For this review, take the finished solid that the model builds, in its own axes (mm). A direction names the side the tool comes from. Coordinates: 2 decimals unless noted, no trailing zeros. Write each loop counter-clockwise with the first axis right and the second up, starting at its lowest first coordinate (ties: lowest second). Pieces come first, ordered by that corner, then holes. Notation, with made-up numbers: (86, -32.75) - (121, -32.75) arc R16 ccw to (121, -26.75) - close; hole circle Ø2 at (39, 82.5). An arc over 180 degrees is marked (long way). Use one line per item in the form item = value. Start each with the question number.
1) For L1, parallel to Y at x = -1.5, z = 5.5; L2, parallel to X at y = 6.25, z = 32; L3, parallel to Y at x = 8, z = 9, list the stretches that pass through material, from the lowest coordinate up. Write a range as from..to.
2) Insertion check: P1, Ø10.5, axis at x = -17.5, z = 12.5, coming from the -Y side; P2, Ø4, axis at x = -37.5, y = 2.5, coming from the -Z side; P3, Ø10, axis at x = -35.5, z = 8.5, coming from the -Y side. Each pin has a flat end and moves straight along its axis. Give the tip position at first contact, or say it passes through.
3) We need section B-B (x = -9.5). Give the boundary of the cut face in (y, z).
4) We need section A-A (y = 2). Give the boundary of the cut face in (x, z).
5) Mouldability with a two-part tool opening along X and no side actions: class faces 4 (the cylindrical face through (-38.185, -10.06, 17.578)), 5 (the flat face through (-9, 7.62, 18)), 6 (the flat face through (8, -8, 0)) as pulls with the +X half, pulls with the -X half, needs draft (parallel to the pull), parting line crosses it, or undercut.
6) We need section D-D (y = -5.5). Give the boundary of the cut face in (x, z), plus the area to 3 significant figures.
7) We need section C-C (x = 3). Give the boundary of the cut face in (y, z), plus the area to 3 significant figures.
8) Tool access review of faces 1 (the flat face through (-8, -7.62, 18)), 2 (the flat face through (-34, -6.35, 8)), 3 (the flat face through (5.17, 0.11, 17.58)): name each direction out of +Z, -Z, +X, -X, +Y, -Y from which nothing blocks a thin tool from reaching the whole face with its end or side.
```python
from build123d import *

# Parameters (mm, degrees)
F1_DEPTH      = 34.671
F2_R          = 2.54
F5_DEPTH      = 59.1859747542
F7_DEPTH      = 6.35
F7_DEPTH_BACK = 6.35


with BuildPart() as f1:
    # F0 (on Top) → F1 (new body)
    with BuildSketch(Plane.XY):
        Polygon((38.89375, 12.192), (-38.89375, 10.795), (-38.89375, -10.795), (38.89375, -12.192), align=None)
    extrude(amount=F1_DEPTH)

    # F2
    f2_edges = [f1.edges().sort_by_distance(p)[0] for p in [
        (-38.89375, -10.795, 17.3355),
        (-38.89375, 10.795, 17.3355),
        (38.89375, -12.192, 17.3355),
        (38.89375, 12.192, 17.3355),
    ]]
    fillet(f2_edges, radius=F2_R)

    # F4 (on face) → F5 (cut, through all)
    with BuildSketch(Plane(origin=(-15.6927490779, 0, 43.1154737408), x_dir=(0.9396926208, 0, 0.3420201433), z_dir=(0.3420201433, 0, -0.9396926208))):
        with BuildLine():
            Line((10.8700105196, 7.62), (-14.5299894804, 7.62))
            ThreePointArc((-14.5299894804, 7.62), (-22.1499894804, 0), (-14.5299894804, -7.62))
            Line((-14.5299894804, -7.62), (10.8700105196, -7.62))
            Line((10.8700105196, -7.62), (10.8700105196, 7.62))
        make_face()
    extrude(amount=F5_DEPTH, mode=Mode.SUBTRACT)

    # F6 (on Front) → F7 (cut, two sides)
    with BuildSketch(Plane.XZ) as f7_sk:
        Polygon((-36.3993589719, 0), (-26.2745380078, 0), (-33.670413168, 20.32), (-38.89375, 20.32), (-38.89375, 0), align=None)
    extrude(amount=-F7_DEPTH, mode=Mode.SUBTRACT)
    extrude(f7_sk.sketch, amount=F7_DEPTH_BACK, mode=Mode.SUBTRACT)


solid = f1.part
```
Determined:
q1.L1 = -11.47..-7.62, 7.62..11.47
q1.L2 = -38.89..-31.75, -0.08..38.89
q1.L3 = -11.64..-7.62, 7.62..11.64
q2.P1 = -11.27
q2.P2 = 20.32
q2.P3 = -10.95
q3.outline = (-11.32, 0) - (-7.62, 0) - (-7.62, 34.67) - (-11.32, 34.67) - close; (7.62, 0) - (11.32, 0) - (11.32, 34.67) - (7.62, 34.67) - close
q4.outline = (-38.89, 20.32) - (-33.67, 20.32) - (-26.27, 0) - (-23.29, 0) - (-35.91, 34.67) - (-38.89, 34.67) - close; (-1.05, 34.67) - (11.57, 0) - (38.89, 0) - (38.89, 34.67) - close
q5.face_4 = pulls with the -X half
q5.face_5 = undercut
q5.face_6 = needs draft
q6.outline = (-38.89, 20.32) - (-33.67, 20.32) - (-26.27, 0) - (-21.07, 0) - (-33.69, 34.67) - (-38.89, 34.67) - close; (-1.05, 34.67) - (11.57, 0) - (38.89, 0) - (38.89, 34.67) - close
q6.area = 1,380 mm²
q7.outline = (-11.55, 0) - (-7.62, 0) - (-7.62, 23.54) - (7.62, 23.54) - (7.62, 0) - (11.55, 0) - (11.55, 34.67) - (-11.55, 34.67) - close
q7.area = 442 mm²
q8.face_1 = none
q8.face_2 = -Z, -X
q8.face_3 = -Z
